For this review, take the finished solid that the model builds, in its own axes (mm). Face numbers are marked on the shaded views. Give positions to 0.01 mm unless a question says otherwise; leave off trailing zeros. Use CSV: the item, a comma, the result in double quotes. Start each with the question number.
1. Insertion check: P1, Ø1.5, axis at x = -81.5, y = 13, coming from the -Z side; P2, Ø11, axis at x = -44, y = 6.5, coming from the -Z side; P3, Ø4, axis at y = 4, z = 11.5, coming from the -X side; P4, Ø5, axis at x = 72.5, z = 0, coming from the -Y side. Each pin has a flat end and moves straight along its axis. Give the tip position at first contact, or say it passes through.
2. Take a section at A-A, the plane z = 18. State how many separate pieces and enclosed holes the cut face has, and give its area (3 significant figures).
3. To check wall thickness, follow line 1 (X direction, y = 12.5, z = -1); line 2 (Z direction, x = 27, y = 20); line 3 (Z direction, x = 14.5, y = 4.5). State the ranges of each line that lie inside material, in increasing order. Write a range as [from, to].
4. The part is to be moulded in two halves that separate along X. For the marked faces 1, 2 and 3, say which applies: pulls with the +X half, pulls with the -X half, needs draft (parallel to the pull), parting line crosses it, or undercut.
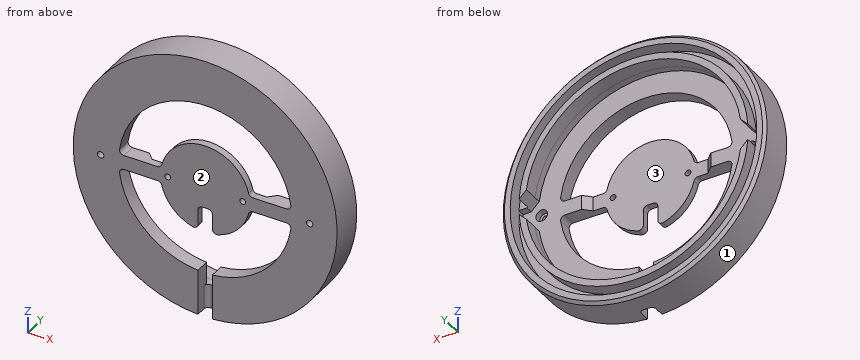
from build123d import *

# Parameters (mm, degrees)
SKETCH1_R                                           = 91.5
BOSS_EXTRUDE1_DEPTH                                 = 10
CUT_EXTRUDE1_DEPTH                                  = 130.78636292
SKETCH3_R                                           = 40
CUT_EXTRUDE2_DEPTH                                  = 5
SKETCH4_R                                           = 91.5
SKETCH4_R_2                                         = 75
BOSS_EXTRUDE2_DEPTH                                 = 5
SKETCH5_R                                           = 91.5
SKETCH5_R_2                                         = 85.5
BOSS_EXTRUDE3_DEPTH                                 = 10
CHAMFER1_SIZE                                       = 2
F_4_5_4_5_DIAMETER_HOLE1_D                          = 4.5
CUT_EXTRUDE3_DEPTH                                  = 91
FILLET1_R                                           = 3
CHAMFER2_SIZE                                       = 5
CHAMFER3_SIZE                                       = 5
SKETCH10_W                                          = 10
SKETCH10_H                                          = 20
CUT_EXTRUDE4_DEPTH                                  = 91
FILLET2_R                                           = 3
FILLET3_R                                           = 3
BOSS_EXTRUDE4_DEPTH                                 = 10
SKETCH12_W                                          = 10
SKETCH12_H                                          = 35
CUT_EXTRUDE5_DEPTH                                  = 10
FILLET4_R                                           = 3
SKETCH13_R                                          = 2
CUT_EXTRUDE6_DEPTH                                  = 10
CBORE_FOR_M4_HEX_SOCKET_HEAD_CAP_SCREW1_D           = 4.5
CBORE_FOR_M4_HEX_SOCKET_HEAD_CAP_SCREW1_CBORE_D     = 8
CBORE_FOR_M4_HEX_SOCKET_HEAD_CAP_SCREW1_CBORE_DEPTH = 4.4


# Some blends are built 0.0001 mm under size
with BuildPart() as part:
    # Sketch1 → Boss-Extrude1 (new body)
    with BuildSketch(Plane(origin=(0, 0, 0), x_dir=(1, 0, 0), z_dir=(0, 1, 0))):
        with Locations(Location((0, 0, 0), (0, 0, 270))):
            Circle(SKETCH1_R)
    extrude(amount=BOSS_EXTRUDE1_DEPTH)

    # Sketch2 → Cut-Extrude1 (cut, through all)
    with BuildSketch(Plane(origin=(0, 10, 0), x_dir=(1, 0, 0), z_dir=(0, 1, 0))):
        with BuildLine():
            ThreePointArc((59.791303716, 5), (0, 60), (-59.791303716, 5))
            Line((-59.791303716, 5), (-30.594117082, 5))
            ThreePointArc((-30.594117082, 5), (0, 31), (30.594117082, 5))
            Line((30.594117082, 5), (59.791303716, 5))
        make_face()
        with BuildLine():
            Line((-30.594117082, -5), (-59.791303716, -5))
            ThreePointArc((-59.791303716, -5), (0, -60), (59.791303716, -5))
            Line((59.791303716, -5), (30.594117082, -5))
            ThreePointArc((30.594117082, -5), (0, -31), (-30.594117082, -5))
        make_face()
    extrude(amount=-CUT_EXTRUDE1_DEPTH, mode=Mode.SUBTRACT)

    # Sketch3 → Cut-Extrude2 (cut)
    with BuildSketch(Plane(origin=(0, 10, 0), x_dir=(1, 0, 0), z_dir=(0, 1, 0))):
        Circle(SKETCH3_R)
    extrude(amount=-CUT_EXTRUDE2_DEPTH, mode=Mode.SUBTRACT)

    # Sketch4 → Boss-Extrude2 (add)
    with BuildSketch(Plane(origin=(0, 10, 0), x_dir=(1, 0, 0), z_dir=(0, 1, 0))):
        with Locations(Location((0, 0, 0), (0, 0, 270))):
            Circle(SKETCH4_R)
        with Locations(Location((0, 0, 0), (0, 0, 270))):
            Circle(SKETCH4_R_2, mode=Mode.SUBTRACT)
    extrude(amount=BOSS_EXTRUDE2_DEPTH)

    # Sketch5 → Boss-Extrude3 (add)
    with BuildSketch(Plane(origin=(0, 15, 0), x_dir=(1, 0, 0), z_dir=(0, 1, 0))):
        with Locations(Location((0, 0, 0), (0, 0, 270))):
            Circle(SKETCH5_R)
        with Locations(Location((0, 0, 0), (0, 0, 270))):
            Circle(SKETCH5_R_2, mode=Mode.SUBTRACT)
    extrude(amount=BOSS_EXTRUDE3_DEPTH)

    # Chamfer1
    chamfer1_edges = [part.edges().sort_by_distance(p)[0] for p in [
        (0, 25, -91.5),
    ]]
    chamfer(chamfer1_edges, length=CHAMFER1_SIZE)

    # Ø4.5 (4.5) Diameter Hole1 (through all)
    with Locations(Plane(origin=(0, 10, 0), x_dir=(1, 0, 0), z_dir=(0, 1, 0))):
        with Locations((-72.5, 0), (72.5, 0)):
            Hole(F_4_5_4_5_DIAMETER_HOLE1_D / 2)

    # Sketch9 → Cut-Extrude3 (cut)
    with BuildSketch(Plane(origin=(0, 10, 0), x_dir=(1, 0, 0), z_dir=(0, 1, 0))):
        with BuildLine():
            Line((-85.353675961, 5), (85.353675961, 5))
            ThreePointArc((85.353675961, 5), (85.5, 0), (85.353675961, -5))
            Line((85.353675961, -5), (-85.353675961, -5))
            ThreePointArc((-85.353675961, -5), (-85.5, 0), (-85.353675961, 5))
        make_face()
    extrude(amount=CUT_EXTRUDE3_DEPTH, mode=Mode.SUBTRACT)

    # Fillet1
    fillet1_edges = [part.edges().sort_by_distance(p)[0] for p in [
        (-59.791303716, 5, -5),
        (59.791303716, 5, -5),
        (59.791303716, 5, 5),
        (-59.791303716, 5, 5),
    ]]
    fillet(fillet1_edges, radius=FILLET1_R)

    # Chamfer2
    chamfer2_edges = [part.edges().sort_by_distance(p)[0] for p in [
        (-40, 10, 0),
        (40, 10, 0),
    ]]
    chamfer(chamfer2_edges, length=CHAMFER2_SIZE - 0.0001)  # a hair under: the kernel refuses the full size

    # Chamfer3
    # the kernel refuses this chamfer: 5.369942673, 5 mm, written as the material it takes off along each edge
    with BuildSketch(Plane(origin=(-74.833147735, 29.456298598, -5), x_dir=(0.10396392346922531, 0, -0.9945810689013164), z_dir=(0, -1, 0))) as chamfer3_piece_1:
        with BuildLine():
            Line((5.614084599, 0), (-CHAMFER3_SIZE * 0.103963923469, -CHAMFER3_SIZE * 0.994581068901))
            Line((-CHAMFER3_SIZE * 0.103963923469, -CHAMFER3_SIZE * 0.994581068901), (0, 0))
            ThreePointArc((0, 0), (2.890602355, -0.05250177), (5.614084599, 0))
        make_face()
    extrude(amount=19.456298598, mode=Mode.SUBTRACT)
    with BuildSketch(Plane(origin=(-74.833147735, 29.456298598, 5), x_dir=(-1, 0, 0), z_dir=(0, -1, 0)), Plane(origin=(74.833147735, 29.456298598, -5), x_dir=(1, 0, 0), z_dir=(0, -1, 0))) as chamfer3_piece_2:
        with BuildLine():
            Line((CHAMFER3_SIZE, 0), (-0.583662262, -5.583662262))
            ThreePointArc((-0.583662262, -5.583662262), (-0.248301095, -2.88039667), (0, 0))
            Line((0, 0), (CHAMFER3_SIZE, 0))
        make_face()
    extrude(amount=19.456298598, mode=Mode.SUBTRACT)
    with BuildSketch(Plane(origin=(74.833147735, 29.456298598, 5), x_dir=(1, 0, 0), z_dir=(0, -1, 0))) as chamfer3_piece_3:
        with BuildLine():
            Line((CHAMFER3_SIZE, 0), (-0.583662262, 5.583662262))
            ThreePointArc((-0.583662262, 5.583662262), (-0.248301095, 2.88039667), (0, 0))
            Line((0, 0), (CHAMFER3_SIZE, 0))
        make_face()
    extrude(amount=19.456298598, mode=Mode.SUBTRACT)

    # Sketch10 → Cut-Extrude4 (cut)
    with BuildSketch(Plane.XY.offset(-40)):
        Rectangle(SKETCH10_W, SKETCH10_H)
    extrude(amount=-CUT_EXTRUDE4_DEPTH, mode=Mode.SUBTRACT)

    # Fillet2
    fillet2_edges = [part.edges().sort_by_distance(p)[0] for p in [
        (5, 10, -83.098216789),
        (-5, 10, -83.098216789),
    ]]
    fillet(fillet2_edges, radius=FILLET2_R)

    # Fillet3
    fillet3_edges = [part.edges().sort_by_distance(p)[0] for p in [
        (-30.594117082, 2.5, -5),
        (-30.594117082, 2.5, 5),
        (30.594117082, 2.5, 5),
        (30.594117082, 2.5, -5),
    ]]
    fillet(fillet3_edges, radius=FILLET3_R)

    # Sketch11 → Boss-Extrude4 (add)
    with BuildSketch(Plane(origin=(0, 15, 0), x_dir=(1, 0, 0), z_dir=(0, 1, 0))):
        with BuildLine():
            Line((-74.249485474, 10.583662262), (-79.307755217, 5.525392519))
            ThreePointArc((-79.307755217, 5.525392519), (0, 79.5), (79.307755217, 5.525392519))
            Line((79.307755217, 5.525392519), (74.249485474, 10.583662262))
            ThreePointArc((74.249485474, 10.583662262), (0, 75), (-74.249485474, 10.583662262))
        make_face()
        with BuildLine():
            Line((-74.249485474, -10.583662262), (-79.307755217, -5.525392519))
            ThreePointArc((-79.307755217, -5.525392519), (0, -79.5), (79.307755217, -5.525392519))
            Line((79.307755217, -5.525392519), (74.249485474, -10.583662262))
            ThreePointArc((74.249485474, -10.583662262), (0, -75), (-74.249485474, -10.583662262))
        make_face()
    extrude(amount=BOSS_EXTRUDE4_DEPTH)

    # Sketch12 → Cut-Extrude5 (cut)
    with BuildSketch(Plane(origin=(0, 5, 0), x_dir=(1, 0, 0), z_dir=(0, 1, 0))):
        with Locations((0, 31)):
            Rectangle(SKETCH12_W, SKETCH12_H)
    extrude(amount=-CUT_EXTRUDE5_DEPTH, mode=Mode.SUBTRACT)

    # Fillet4
    fillet4_edges = [part.edges().sort_by_distance(p)[0] for p in [
        (5, 2.5, -30.594117082),
        (5, 2.5, -13.5),
        (-5, 2.5, -30.594117082),
        (-5, 2.5, -13.5),
    ]]
    fillet(fillet4_edges, radius=FILLET4_R)

    # Sketch13 → Cut-Extrude6 (cut)
    with BuildSketch(Plane(origin=(0, 0, 0), x_dir=(-1, 0, 0), z_dir=(0, -1, 0))):
        with Locations(Location((26, 0, 0), (0, 0, 90))):
            Circle(SKETCH13_R)
        with Locations(Location((-26, 0, 0), (0, 0, 90))):
            Circle(SKETCH13_R)
    extrude(amount=-CUT_EXTRUDE6_DEPTH, mode=Mode.SUBTRACT)

    # CBORE for M4 Hex Socket Head Cap Screw1 (through all)
    with Locations(Plane(origin=(0, 10, 0), x_dir=(1, 0, 0), z_dir=(0, 1, 0))):
        with Locations((-72.5, 0), (72.5, 0)):
            CounterBoreHole(CBORE_FOR_M4_HEX_SOCKET_HEAD_CAP_SCREW1_D / 2, CBORE_FOR_M4_HEX_SOCKET_HEAD_CAP_SCREW1_CBORE_D / 2, CBORE_FOR_M4_HEX_SOCKET_HEAD_CAP_SCREW1_CBORE_DEPTH)


solid = part.part
Result set:
1,P1,"z = -43.03"
1,P2,"z = -83.01"
1,P3,"x = -91.01"
1,P4,"y = 0"
2,separate pieces,"3"
2,enclosed holes,"0"
2,area,"1,280 mm2"
3,line 1,"[-91.49, -85.49], [85.49, 91.49]"
3,line 2,"[-87.43, -81.12], [-74.77, -69.97], [69.97, 74.77], [81.12, 87.43]"
3,line 3,"[-90.34, -58.22], [-27.4, 27.4], [58.22, 90.34]"
4,face 1,"parting line crosses it"
4,face 2,"needs draft"
4,face 3,"undercut"
